The model under review builds one solid part; all positions refer to its coordinate system, in mm. A direction names the side the tool comes from. Give positions to 0.01 mm unless a question says otherwise; leave off trailing zeros.
from build123d import *

# Parameters (mm, degrees)
SKETCH1_W           = 65.0875
SKETCH1_H           = 31.75
BOSS_EXTRUDE1_DEPTH = 4.7625
CUT_EXTRUDE1_DEPTH  = 38.441112618
SKETCH3_R           = 1.905
CUT_EXTRUDE2_DEPTH  = 12.7
SKETCH4_R           = 1.905
CUT_EXTRUDE3_DEPTH  = 38.441112618
CUT_EXTRUDE4_DEPTH  = 38.441112618
FILLET3_R           = 3.175
FILLET6_R           = 12.7
FILLET5_R           = 1.5875


# Some blends are built 0.0001 mm under size
with BuildPart() as part:
    # Sketch1 → Boss-Extrude1 (new, symmetric)
    with BuildSketch(Plane.XY):
        Rectangle(SKETCH1_W, SKETCH1_H)
    extrude(amount=BOSS_EXTRUDE1_DEPTH, both=True)

    # Sketch2 → Cut-Extrude1 (cut, through all)
    with BuildSketch(Plane.XY.offset(4.7625)):
        Polygon((-23.01875, -15.875), (-12.7, -6.35), (12.7, -6.35), (23.01875, -15.875), align=None)
    extrude(amount=-CUT_EXTRUDE1_DEPTH, mode=Mode.SUBTRACT)

    # Sketch3 → Cut-Extrude2 (cut)
    with BuildSketch(Plane(origin=(32.54375, 0, 0), x_dir=(0, 0, -1), z_dir=(1, 0, 0))):
        with Locations((0, 11.1125)):
            Circle(SKETCH3_R)
        with Locations((0, -11.1125)):
            Circle(SKETCH3_R)
    cut_extrude2 = extrude(amount=-CUT_EXTRUDE2_DEPTH, mode=Mode.SUBTRACT)

    # Mirror2: Cut-Extrude2 across plane
    add(cut_extrude2.mirror(Plane(origin=(0, 0, 0), x_dir=(0, 0, 1), z_dir=(1, 0, 0))), mode=Mode.SUBTRACT)

    # Sketch4 → Cut-Extrude3 (cut, through all)
    with BuildSketch(Plane(origin=(0, 0, -4.7625), x_dir=(-1, 0, 0), z_dir=(0, 0, -1))):
        with Locations((-19.05, 0)):
            Circle(SKETCH4_R)
        with Locations((19.05, 0)):
            Circle(SKETCH4_R)
    extrude(amount=-CUT_EXTRUDE3_DEPTH, mode=Mode.SUBTRACT)

    # Sketch5 → Cut-Extrude4 (cut, through all)
    with BuildSketch(Plane(origin=(0, 0, -4.7625), x_dir=(-1, 0, 0), z_dir=(0, 0, -1))):
        with BuildLine():
            Line((-14.224417781, -1.5875), (14.224417781, -1.5875))
            ThreePointArc((14.224417781, -1.5875), (14.515266075, 2.289669895), (17.4625, 4.825582219))
            Line((17.4625, 4.825582219), (17.4625, 12.7))
            Line((17.4625, 12.7), (-17.4625, 12.7))
            Line((-17.4625, 12.7), (-17.4625, 4.825582219))
            ThreePointArc((-17.4625, 4.825582219), (-14.515266075, 2.289669895), (-14.224417781, -1.5875))
        make_face()
    extrude(amount=-CUT_EXTRUDE4_DEPTH, mode=Mode.SUBTRACT)

    # Fillet3
    fillet3_edges = [part.edges().sort_by_distance(p)[0] for p in [
        (-17.4625, 4.825582219, 0),
        (-14.224417781, -1.5875, 0),
        (14.224417781, -1.5875, 0),
        (17.4625, 4.825582219, 0),
        (17.4625, 12.7, 0),
        (-17.4625, 12.7, 0),
    ]]
    fillet(fillet3_edges, radius=FILLET3_R)

    # Fillet6
    # the kernel refuses this fillet: 12.7 mm, written as the material it adds along each edge
    with BuildSketch(Plane(origin=(-12.7, -6.35, 4.7625), x_dir=(-0.7348034446274875, -0.6782801027330664, 0), z_dir=(0, 0, -1)), Plane(origin=(12.7, -6.35, 4.7625), x_dir=(-1, 0, 0), z_dir=(0, 0, -1))) as fillet6_piece_1:
        with BuildLine():
            CenterArc((FILLET6_R * 0.390983834413, -FILLET6_R), FILLET6_R, 90, 42.709389957)
            Line((-FILLET6_R * 0.28729626832, -FILLET6_R * 0.265196555373), (0, 0))
            Line((0, 0), (FILLET6_R * 0.390983834413, 0))
        make_face()
    extrude(amount=9.525)
    # the kernel refuses this fillet: 12.7 mm, written as the material it takes off along each edge
    with BuildSketch(Plane(origin=(23.01875, -15.875, 17.176236743), x_dir=(1, 0, 0), z_dir=(0, 0, -1))) as fillet6_2_piece_1:
        with BuildLine():
            CenterArc((FILLET6_R * 0.390983834413, -FILLET6_R), FILLET6_R, 90, 42.709389957)
            Line((-FILLET6_R * 0.28729626832, -FILLET6_R * 0.265196555373), (0, 0))
            Line((0, 0), (FILLET6_R * 0.390983834413, 0))
        make_face()
    extrude(amount=34.352473485, mode=Mode.SUBTRACT)
    with BuildSketch(Plane(origin=(-23.01875, -15.875, 17.176236743), x_dir=(-1, 0, 0), z_dir=(0, 0, -1))) as fillet6_2_piece_2:
        with BuildLine():
            CenterArc((FILLET6_R * 0.390983834413, FILLET6_R), FILLET6_R, 227.290610043, 42.709389957)
            Line((-FILLET6_R * 0.28729626832, FILLET6_R * 0.265196555373), (0, 0))
            Line((0, 0), (FILLET6_R * 0.390983834413, 0))
        make_face()
    extrude(amount=34.352473485, mode=Mode.SUBTRACT)

    # Fillet5
    fillet5_edges = [part.edges().sort_by_distance(p)[0] for p in [
        (0, -1.5875, 4.7625),
        (-16.53256403, 11.77006403, -4.7625),
        (-16.53256403, 11.77006403, 4.7625),
        (-17.106752578, 5.282383875, -4.7625),
        (-17.106752578, 5.282383875, 4.7625),
        (17.106752578, 5.282383875, -4.7625),
        (17.106752578, 5.282383875, 4.7625),
        (16.53256403, 11.77006403, -4.7625),
        (16.53256403, 11.77006403, 4.7625),
        (12.966759515, -0.863949238, -4.7625),
        (12.966759515, -0.863949238, 4.7625),
        (-12.966759515, -0.863949238, -4.7625),
        (-12.966759515, -0.863949238, 4.7625),
        (-17.859375, -11.1125, 4.7625),
        (0, -6.35, 4.7625),
        (17.859375, -11.1125, 4.7625),
        (30.263997349, -15.875, 4.7625),
        (23.359660801, -15.003069318, 4.7625),
        (-23.359660801, -15.003069318, 4.7625),
        (-17.859375, -11.1125, -4.7625),
        (30.263997349, -15.875, -4.7625),
        (17.859375, -11.1125, -4.7625),
        (0, -6.35, -4.7625),
        (23.359660801, -15.003069318, -4.7625),
        (-23.359660801, -15.003069318, -4.7625),
        (-12.359089199, -7.221930682, 4.7625),
        (-12.359089199, -7.221930682, -4.7625),
        (12.359089199, -7.221930682, 4.7625),
        (12.359089199, -7.221930682, -4.7625),
        (-30.263997349, -15.875, 4.7625),
        (-30.263997349, -15.875, -4.7625),
        (0, 15.875, -4.7625),
        (0, 12.7, -4.7625),
        (0, 12.7, 4.7625),
        (0, 15.875, 4.7625),
        (-17.4625, 8.133835742, -4.7625),
        (-17.4625, 8.133835742, 4.7625),
        (-14.786009483, 2.7613013, -4.7625),
        (-14.786009483, 2.7613013, 4.7625),
        (14.786009483, 2.7613013, -4.7625),
        (14.786009483, 2.7613013, 4.7625),
        (17.4625, 8.133835742, -4.7625),
        (17.4625, 8.133835742, 4.7625),
        (0, -1.5875, -4.7625),
    ]]
    fillet(fillet5_edges, radius=FILLET5_R - 0.0001)  # a hair under: the kernel refuses the full size


solid = part.part
1) To check wall thickness, follow probe 1 along Y at (x, z) = (-30, 0) (1 decimal); probe 2 along Z at (x, y) = (2, 14.5); probe 3 along X at (y, z) = (9, 0.75). State the ranges of each line that lie inside material, in increasing order.
2) The part is to be moulded in two halves that separate along X. For faces 1 (the flat face through (19.844, 11, 0)), 2 (the cylindrical face through (-17.94, 8.11, -4.31)), 3 (the cylindrical face through (26.283, 9.253, 0.413)), say which applies: +X half, -X half, draft (parallel to the pull), parting line (faces both ways), or undercut.
3) Tool access review of faces 4 (the cylindrical face through (17.94, 8.15, -4.31)), 5 (the cylindrical face through (17.097, 5.264, 0.044)), 6 (the cylindrical face through (0.108, -5.897, 4.285)), 7 (the flat face through (-19.844, 11, 0)), 8 (the cylindrical face through (12.3, -7.2, 0)): name each direction out of +Z, -Z, +X, -X, +Y, -Y from which nothing blocks a thin tool from reaching the whole face with its end or side.
4) Insertion check: pin 1 (3 mm diameter, centred on x = -2.5, z = 0, fed in from -Y); pin 2 (4 mm diameter, centred on x = 13.5, z = 2, fed in from -Y); pin 3 (1.9 mm diameter, centred on y = 11.5, z = -0.5, fed in from +X); pin 4 (3 mm diameter, centred on y = -11.5, z = -1, fed in from -X). Each pin has a flat end and moves straight along its axis. Give the tip position at first contact, or say it passes through.
5) Consider section B-B, the plane z = 0. State how many separate pieces and enclosed holes the cut face has, then the cut area to 3 significant figures.
Answer block:
1. probe 1: y = -15.9 to -13, -9.2 to 9.2, 13 to 15.9
1. probe 2: z = -4.75 to 4.75
1. probe 3: x = -32.54 to -17.46, 17.46 to 32.54
2. face 1: +X half
2. face 2: undercut
2. face 3: draft
3. face 4: -Z
3. face 5: +Z, -Z
3. face 6: +Z, -Y
3. face 7: -X
3. face 8: +Z, -Z, -Y
4. pin 1: stops at y = -6.35
4. pin 2: stops at y = -9
4. pin 3: stops at x = 19.84
4. pin 4: stops at x = -32.54
5. separate pieces: 3
5. enclosed holes: 3
5. area: 1,060 mm2
